For this review, take the finished solid that the model builds, in its own axes (mm). Face numbers are marked on the shaded views. A direction names the side the tool comes from. Coordinates: 2 decimals unless noted, no trailing zeros. Write each loop counter-clockwise with the first axis right and the second up, starting at its lowest first coordinate (ties: lowest second). Pieces come first, ordered by that corner, then holes.
```python
from build123d import *

# Parameters (mm, degrees)
SKETCH1_W           = 86
SKETCH1_H           = 40
BOSS_EXTRUDE1_DEPTH = 12
SKETCH2_W           = 15.5
SKETCH2_H           = 40
BOSS_EXTRUDE2_DEPTH = 50
SKETCH3_R           = 7.25
CUT_EXTRUDE1_DEPTH  = 50
FILLET1_R           = 15
SKETCH5_R           = 2
CUT_EXTRUDE2_DEPTH  = 50
CHAMFER1_SIZE       = 2
SKETCH6_R           = 3
CUT_EXTRUDE3_DEPTH  = 10
SKETCH7_R           = 5
CUT_EXTRUDE4_DEPTH  = 5


with BuildPart() as part:
    # Sketch1 → Boss-Extrude1 (new body)
    with BuildSketch(Plane.XY):
        with Locations((43, 20)):
            Rectangle(SKETCH1_W, SKETCH1_H)
    extrude(amount=BOSS_EXTRUDE1_DEPTH)

    # Sketch2 → Boss-Extrude2 (add)
    with BuildSketch(Plane.XY.offset(12)):
        with Locations((25.75, 20)):
            Rectangle(SKETCH2_W, SKETCH2_H)
        with Locations((60.25, 20)):
            Rectangle(SKETCH2_W, SKETCH2_H)
    extrude(amount=BOSS_EXTRUDE2_DEPTH)

    # Sketch3 → Cut-Extrude1 (cut)
    with BuildSketch(Plane.ZY.offset(-18)):
        with Locations(Location((37, 20, 0), (0, 0, 270))):
            Circle(SKETCH3_R)
    extrude(amount=-CUT_EXTRUDE1_DEPTH, mode=Mode.SUBTRACT)

    # Fillet1
    fillet1_edges = [part.edges().sort_by_distance(p)[0] for p in [
        (25.75, 0, 62),
        (25.75, 40, 62),
        (60.25, 0, 62),
        (60.25, 40, 62),
    ]]
    fillet(fillet1_edges, radius=FILLET1_R)

    # Sketch5 → Cut-Extrude2 (cut)
    with BuildSketch(Plane.XY.offset(12)):
        with Locations((9, 30)):
            Circle(SKETCH5_R)
        with Locations((9, 10)):
            Circle(SKETCH5_R)
        with Locations((43, 30)):
            Circle(SKETCH5_R)
        with Locations((43, 10)):
            Circle(SKETCH5_R)
        with Locations((77, 30)):
            Circle(SKETCH5_R)
        with Locations((77, 10)):
            Circle(SKETCH5_R)
    extrude(amount=-CUT_EXTRUDE2_DEPTH, mode=Mode.SUBTRACT)

    # Chamfer1
    chamfer1_edges = [part.edges().sort_by_distance(p)[0] for p in [
        (7, 30, 12),
        (75, 10, 12),
        (75, 30, 12),
        (41, 10, 12),
        (41, 30, 12),
        (7, 10, 12),
    ]]
    chamfer(chamfer1_edges, length=CHAMFER1_SIZE)

    # Sketch6 → Cut-Extrude3 (cut)
    with BuildSketch(Plane(origin=(0, 0, 0), x_dir=(-1, 0, 0), z_dir=(0, 0, -1))):
        with Locations((-10, 20)):
            Circle(SKETCH6_R)
        with Locations((-40, 20)):
            Circle(SKETCH6_R)
    extrude(amount=-CUT_EXTRUDE3_DEPTH, mode=Mode.SUBTRACT)

    # Sketch7 → Cut-Extrude4 (cut)
    with BuildSketch(Plane(origin=(0, 0, 0), x_dir=(-1, 0, 0), z_dir=(0, 0, -1))):
        with Locations((-10, 20)):
            Circle(SKETCH7_R)
        with Locations((-40, 20)):
            Circle(SKETCH7_R)
    extrude(amount=-CUT_EXTRUDE4_DEPTH, mode=Mode.SUBTRACT)


solid = part.part
```
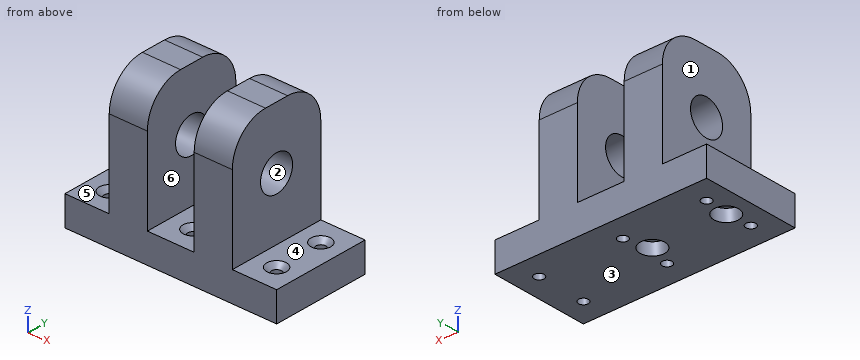
1) The part is to be moulded in two halves that separate along Z. For the marked faces 1, 2 and 3, say which applies: pulls with the +Z half, pulls with the -Z half, needs draft (parallel to the pull), parting line crosses it, or undercut.
2) Clearance check with flat-ended pins moving along their axes: P1, Ø10, axis at x = 41, y = 18, coming from the +Z side; P2, Ø10, axis at y = 18, z = 50.5, coming from the -X side; P3, Ø1, axis at x = 55, z = 51, coming from the -Y side. State where each tip first meets the part, or that it passes through.
3) Consider section D-D (x = 63.5). Give the boundary of the cut face in (y, z).
4) For L1, parallel to X at y = 33, z = 37; L2, parallel to Y at x = 9, z = 7.75; L3, parallel to Z at x = 64, y = 20, list the stretches that pass through material, from the lowest coordinate up.
5) Consider section B-B (x = 77). Give the boundary of the cut face in (y, z), then the cut area to 3 significant figures.
6) Consider section C-C (z = 16.5). Give the boundary of the cut face in (x, y).
7) Consider section A-A (z = 37). Give the boundary of the cut face in (x, y), then the cut area to 4 significant figures.
8) Tool access review of the marked faces 4, 5 and 6: name each direction out of +Z, -Z, +X, -X, +Y, -Y from which nothing blocks a thin tool from reaching the whole face with its end or side.
Results:
1. face 1: needs draft
1. face 2: undercut
1. face 3: pulls with the -Z half
2. P1: stops at z = 12
2. P2: stops at x = 18
2. P3: stops at y = 0.41
3. outline: (0, 0) - (40, 0) - (40, 47) arc R15 ccw to (25, 62) - (15, 62) arc R15 ccw to (0, 47) - close; hole circle Ø14.5 at (20, 37)
4. L1: x = 18 to 33.5, 52.5 to 68
4. L2: y = 0 to 8, 12 to 17.17, 22.83 to 28, 32 to 40
4. L3: z = 0 to 29.75, 44.25 to 62
5. outline: (0, 0) - (8, 0) - (8, 10) - (6, 12) - (0, 12) - close; (12, 0) - (28, 0) - (28, 10) - (26, 12) - (14, 12) - (12, 10) - close; (32, 0) - (40, 0) - (40, 12) - (34, 12) - (32, 10) - close
5. area: 376 mm2
6. outline: (18, 0) - (33.5, 0) - (33.5, 40) - (18, 40) - close; (52.5, 0) - (68, 0) - (68, 40) - (52.5, 40) - close
7. outline: (18, 0) - (33.5, 0) - (33.5, 12.75) - (18, 12.75) - close; (18, 27.25) - (33.5, 27.25) - (33.5, 40) - (18, 40) - close; (52.5, 0) - (68, 0) - (68, 12.75) - (52.5, 12.75) - close; (52.5, 27.25) - (68, 27.25) - (68, 40) - (52.5, 40) - close
7. area: 790.5 mm2
8. face 4: +Z, +X, +Y, -Y
8. face 5: +Z, -X, +Y, -Y
8. face 6: +Z, +Y, -Y
